Autodesk Inventor part; units mm, degrees
ref_plane "YZ Plane" through (0, 0, 0) normal (1, 0, 0) x (0, 1, 0)
ref_plane "XZ Plane" through (0, 0, 0) normal (0, 1, 0) x (-1, 0, 0)
ref_plane "XY Plane" through (0, 0, 0) normal (0, 0, 1) x (1, 0, 0)
sketch "Эскиз1" plane through (0, 0, 0) normal (0, 1, 0) x (-1, 0, 0)
  arc A0 (59.8038, -3) -> (59.8038, 3) centre (65, 0) ccw
  line L0 (29.2568, 0) -> (27.2769, 0)
  circle A1 centre (65, 0) radius 1.45
  line L1 (0, -3) -> (59.8038, -3)
  line L2 (0, 3) -> (59.8038, 3)
  line L3 (0, -9.1238) -> (0, 12.1062) construction
  arc A2 (-59.8038, 3) -> (-59.8038, -3) centre (-65, 0) ccw
  circle A3 centre (-65, 0) radius 1.45
  line L4 (0, -3) -> (-59.8038, -3)
  line L5 (0, 3) -> (-59.8038, 3)
  point P0 (0, 0)
  dimension "d2" = 2.9
  dimension "d5" = 6
  dimension "d7" = 6
  dimension "d8" = 65
extrude "Выдавливание1" add sketch "Эскиз1" along normal mid plane 3
fillet "Сопряжение1" radius 10 4 edges at (-59.8038, 0, -3) (-59.8038, 0, 3) (59.8038, 0, 3) (59.8038, 0, -3)
properties part number "Рычаг головы" material "Золото"
Geometry: final body of the model. Coordinates: model frame, mm. A direction names the side the tool comes from. Give positions to 0.01 mm unless a question says otherwise; leave off trailing zeros. Write each loop counter-clockwise with the first axis right and the second up, starting at its lowest first coordinate (ties: lowest second). Pieces come first, ordered by that corner, then holes. Notation, with made-up numbers: (68, -1) -> (91, -1) arc R17 ccw to (91, 5) -> close; hole circle Ø9 at (-6, -4). An arc over 180 degrees is marked (long way). Answer as a JSON object with one key per item and string values.
1. Cut plane B-B on x = 65. Output: boundary loops of the cut face in (y, z).
Ans:
{"outline": "(-1.5, -6) -> (1.5, -6) -> (1.5, -1.45) -> (-1.5, -1.45) -> close; (-1.5, 1.45) -> (1.5, 1.45) -> (1.5, 6) -> (-1.5, 6) -> close"}
2. Mould query, pull axis X, two halves, no side actions, for faces 4 (the flat face through (1, -1.5, 0)), 5 (the cylindrical face through (-58.8, 0, -3.5)). Classes: pulls with the +X half, pulls with the -X half, needs draft (parallel to the pull), parting line crosses it, or undercut.
Ans:
{"face 4": "needs draft", "face 5": "undercut"}
3. Cut plane C-C on y = 0.55. Output: boundary loops of the cut face in (x, z).
Ans:
{"outline": "(-61.5, -4.88) arc R10 cw to (-55.67, -3) -> (55.67, -3) arc R10 cw to (61.5, -4.88) arc R6 ccw (long way) to (61.5, 4.88) arc R10 cw to (55.67, 3) -> (-55.67, 3) arc R10 cw to (-61.5, 4.88) arc R6 ccw (long way) to start; hole circle Ø2.9 at (-65, 0); hole circle Ø2.9 at (65, 0)"}
4. Cut plane D-D on x = 2. Output: boundary loops of the cut face in (y, z).
Ans:
{"outline": "(-1.5, -3) -> (1.5, -3) -> (1.5, 3) -> (-1.5, 3) -> close"}
5. Access query for faces 1 (the cylindrical face through (-58.693, 0.021, 3.467)), 2 (the cylindrical face through (-71, 0, 0)), 3 (the flat face through (1, 0, -3)). Directions: +Z, -Z, +X, -X, +Y, -Y. A direction counts if a zero-diameter tool reaches every point of the face in a straight line with its end or side. Return the directions, or none.
Ans:
{"face 1": "+Z, +Y, -Y", "face 2": "+Y, -Y", "face 3": "-Z, +Y, -Y"}
6. Contact query for flat-ended pins moving along their axis: pin 1 (2.5 mm diameter, centred on x = -65, z = 0, fed in from -Y); pin 2 (6 mm diameter, centred on x = -32, z = 4, fed in from -Y); pin 3 (1.5 mm diameter, centred on x = 20.5, y = -0.5, fed in from +Z). Output: stop coordinate, or through.
Ans:
{"pin 1": "passes through", "pin 2": "stops at y = -1.5", "pin 3": "stops at z = 3"}
7. Cut plane A-A on z = 0. Output: boundary loops of the cut face in (x, y).
Ans:
{"outline": "(-71, -1.5) -> (-66.45, -1.5) -> (-66.45, 1.5) -> (-71, 1.5) -> close; (-63.55, -1.5) -> (63.55, -1.5) -> (63.55, 1.5) -> (-63.55, 1.5) -> close; (66.45, -1.5) -> (71, -1.5) -> (71, 1.5) -> (66.45, 1.5) -> close"}
8. Ray query, probe 1 along Z at (x, y) = (2, -0.15); probe 2 along X at (y, z) = (-0.5, -5); probe 3 along X at (y, z) = (-1, 4). Return the intervals inside material, ascending. Write a range as from..to.
Ans:
{"probe 1": "z = -3..3", "probe 2": "x = -68.32..-61.68, 61.68..68.32", "probe 3": "x = -69.47..-60.03, 60.03..69.47"}
